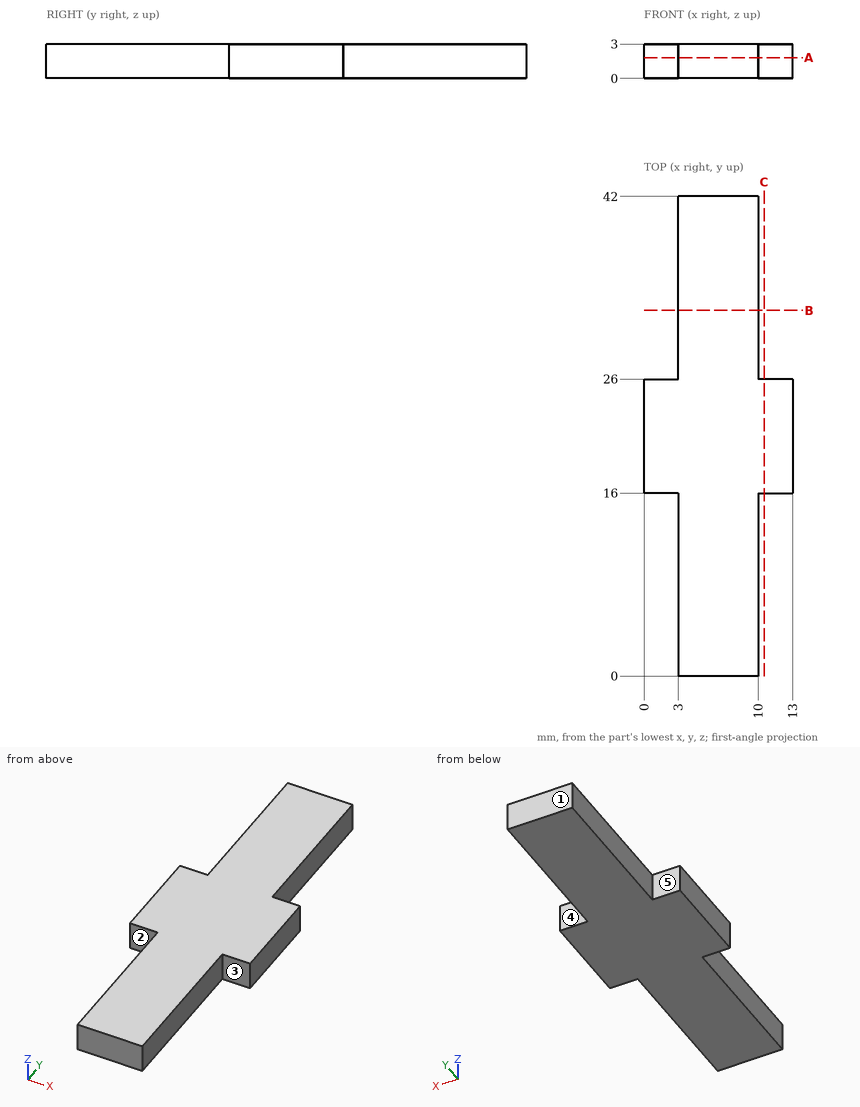
The drawing under review shows one solid part. Ordinate dimensions are in mm from its lowest x, y, z. A direction names the side the tool comes from. Round coordinates to 2 decimals unless told otherwise and drop trailing zeros. Order: outer loops, then holes, each group sorted by start corner. A loop starts at its lowest first (then second) coordinate and runs counter-clockwise, first axis right, second up. Notation, with made-up numbers: (2, 10) -> (45, 10) arc R30 cw to (45, 44) -> close; hole circle Ø2 at (-36.75, 44). An arc over 180 degrees is marked (long way). Return JSON: item names as keys, results as strings.
1. For L1, parallel to X at y = 6.5, z = 0.2; L2, parallel to Y at x = 12, z = 2.55, list the stretches that pass through material, from the lowest coordinate up. Write a range as [from, to].
Answer block:
{"L1": "x = [3, 10]", "L2": "y = [16, 26]"}
2. Take a section at C-C (x = 10.5). Write out the cut boundary in (y, z).
Answer block:
{"outline": "(16, 0) -> (26, 0) -> (26, 3) -> (16, 3) -> close"}
3. Take a section at A-A (z = 1.8). Write out the cut boundary in (x, y).
Answer block:
{"outline": "(0, 16) -> (3, 16) -> (3, 0) -> (10, 0) -> (10, 16) -> (13, 16) -> (13, 26) -> (10, 26) -> (10, 42) -> (3, 42) -> (3, 26) -> (0, 26) -> close"}
4. For the marked faces 1, 2, 3, 4 and 5, list the 3-axis set-ups (+Z, -Z, +X, -X, +Y, -Y) from which the entire face can be reached by the end or side of a thin tool; tool diameter is ignored.
Answer block:
{"face 1": "+Z, -Z, +X, -X, +Y", "face 2": "+Z, -Z, -X, -Y", "face 3": "+Z, -Z, +X, -Y", "face 4": "+Z, -Z, +X, +Y", "face 5": "+Z, -Z, -X, +Y"}
5. Take a section at B-B (y = 32). Write out the cut boundary in (x, z).
Answer block:
{"outline": "(3, 0) -> (10, 0) -> (10, 3) -> (3, 3) -> close"}
6. Insertion check: P1, Ø1.5, axis at x = 2, z = 1, coming from the +Y side; P2, Ø2, axis at x = 4.5, y = 31.5, coming from the -Z side; P3, Ø1.5, axis at y = 30.5, z = 1, coming from the -X side; P4, Ø0.9, axis at y = 36, z = 1.5, coming from the +X side. Each pin has a flat end and moves straight along its axis. Give the tip position at first contact, or say it passes through.
Answer block:
{"P1": "stops at y = 26", "P2": "stops at z = 0", "P3": "stops at x = 3", "P4": "stops at x = 10"}
